For this review, take the finished solid that the model builds, in its own axes (mm). A direction names the side the tool comes from. Round coordinates to 2 decimals unless told otherwise and drop trailing zeros. Loops run counter-clockwise (first coordinate to the right, second up) from the corner with the lowest first, then second, coordinate; pieces in that order, holes last.
1. Consider section D-D on y = -95. State the section outline as (x, z) points.
2. Tool access review of faces 4 (the flat face through (0, -50.664, -19)), 5 (the flat face through (-43, -84, -4.6)), 6 (the cylindrical face through (-0.07, 96.6, -11.75)): name each direction out of +Z, -Z, +X, -X, +Y, -Y from which nothing blocks a thin tool from reaching the whole face with its end or side.
3. Consider section C-C on x = -26. State the section outline as (y, z) points, then the cut area to 3 significant figures.
4. Draft analysis for pull direction Y (two halves, no side actions). For faces 1 (the flat face through (42, -84, -4.6)), 2 (the flat face through (37, -50.664, -11)), 3 (the cylindrical face through (-55.85, -89.61, -9.67)), state which applies: released by +Y, released by -Y, zero draft, split by the parting line, or undercut.
5. Clearance check with flat-ended pins moving along their axes: pin 1 Ø19.5 at (x, y) = (50.5, -88) entering from +Z; pin 2 Ø5 at (y, z) = (36.5, 37.5) entering from +X; pin 3 Ø6 at (y, z) = (15, 5.5) entering from -X. State where each tip first meets the part, or that it passes through.
6. To check wall thickness, follow line 1 along X through (y, z) = (12, -31); line 2 along Y through (x, z) = (55, -7.25); line 3 along Z through (x, y) = (-14, -52). State the ranges of each line that lie inside material, in increasing order.
7. Consider section A-A on x = -55. State the section outline as (y, z) points, then the cut area to 3 significant figures.
8. Consider section B-B on z = -8. State the section outline as (x, y) points, then the cut area to 3 significant figures.
from build123d import *

# Parameters (mm, degrees)
F0_R     = 9.5
F1_DEPTH = 5
F2_R     = 6.5
F2_W     = 10
F2_H     = 65
F3_DEPTH = 10
F4_R     = 5


with BuildPart() as f1:
    # F0 (on Right) → F1 (new body, symmetric)
    with BuildSketch(Plane.YZ):
        Polygon((-115.6638563656, 25.4), (-115.6638563656, -14.6), (-50.6638563656, -14.6), (-50.6638563656, -24.125), (-0.6638563656, -44.6), (109.3361436344, -44.6), (109.3361436344, 20.4), (-10.6638563656, 55.4), (-85.6638563656, 55.4), align=None)
        with Locations((87.5361436344, -14.6)):
            Circle(F0_R, mode=Mode.SUBTRACT)
    extrude(amount=F1_DEPTH, both=True)

    # F2 (on face) → F3 (join)
    with BuildSketch(Plane(origin=(0, 0, -14.6), x_dir=(1, 0, 0), z_dir=(0, 0, -1))):
        with BuildLine():
            ThreePointArc((-75, 55.6638563656), (-73.5355339059, 52.1283224597), (-70, 50.6638563656))
            Line((-70, 50.6638563656), (-5, 50.6638563656))
            Line((-5, 50.6638563656), (-5, 115.6638563656))
            Line((-5, 115.6638563656), (-70, 115.6638563656))
            ThreePointArc((-70, 115.6638563656), (-73.5355339059, 114.1993902716), (-75, 110.6638563656))
            Line((-75, 110.6638563656), (-75, 55.6638563656))
        make_face()
        with Locations((-55, 83.1638563656)):
            Circle(F2_R, mode=Mode.SUBTRACT)
        with Locations((0, 83.1638563656)):
            Rectangle(F2_W, F2_H)
        with BuildLine():
            Line((5, 115.6638563656), (5, 50.6638563656))
            Line((5, 50.6638563656), (70, 50.6638563656))
            ThreePointArc((70, 50.6638563656), (73.5355339059, 52.1283224597), (75, 55.6638563656))
            Line((75, 55.6638563656), (75, 110.6638563656))
            ThreePointArc((75, 110.6638563656), (73.5355339059, 114.1993902716), (70, 115.6638563656))
            Line((70, 115.6638563656), (5, 115.6638563656))
        make_face()
        with Locations((55, 83.1638563656)):
            Circle(F2_R, mode=Mode.SUBTRACT)
    extrude(amount=-F3_DEPTH)

    # F4
    f4_edges = [f1.edges().sort_by_distance(p)[0] for p in [
        (5, -83.163856, -4.6),
        (-5, -83.163856, -4.6),
    ]]
    fillet(f4_edges, radius=F4_R)


solid = f1.part
Resolved:
1. outline: (-75, -14.6) - (75, -14.6) - (75, -4.6) - (10, -4.6) arc R5 cw to (5, 0.4) - (5, 46.06) - (-5, 46.06) - (-5, 0.4) arc R5 cw to (-10, -4.6) - (-75, -4.6) - close
2. face 4: -Z, +X, -X, -Y
2. face 5: +Z, -X, +Y, -Y
2. face 6: +X, -X
3. outline: (-115.66, -14.6) - (-50.66, -14.6) - (-50.66, -4.6) - (-115.66, -4.6) - close
3. area: 650 mm2
4. face 1: zero draft
4. face 2: released by +Y
4. face 3: undercut
5. pin 1: stops at z = -4.6
5. pin 2: stops at x = 5
5. pin 3: stops at x = -5
6. line 1: x = -5 to 5
6. line 2: y = -115.66 to -89.66, -76.66 to -50.66
6. line 3: z = -14.6 to -4.6
7. outline: (-115.66, -14.6) - (-89.66, -14.6) - (-89.66, -4.6) - (-115.66, -4.6) - close; (-76.66, -14.6) - (-50.66, -14.6) - (-50.66, -4.6) - (-76.66, -4.6) - close
7. area: 520 mm2
8. outline: (-75, -110.66) arc R5 ccw to (-70, -115.66) - (70, -115.66) arc R5 ccw to (75, -110.66) - (75, -55.66) arc R5 ccw to (70, -50.66) - (5, -50.66) - (5, 80.7) - (-5, 80.7) - (-5, -50.66) - (-70, -50.66) arc R5 ccw to (-75, -55.66) - close; (-5, 94.37) - (5, 94.37) - (5, 109.34) - (-5, 109.34) - close; hole circle Ø13 at (-55, -83.16); hole circle Ø13 at (55, -83.16)
8. area: 10,900 mm2
